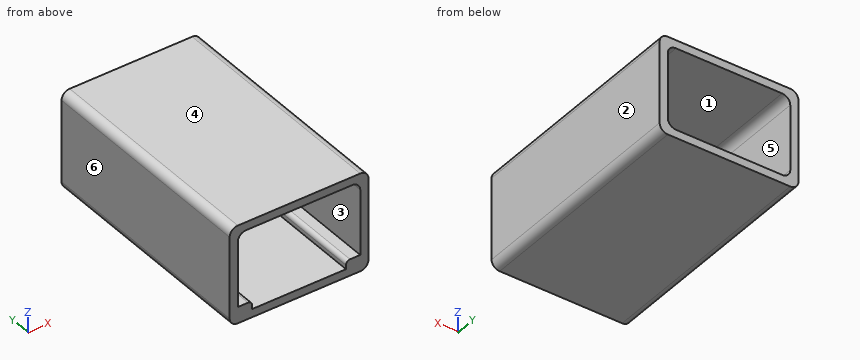
from build123d import *

# Parameters (mm, degrees)
BOSS_EXTRUDE4_DEPTH = 57
BOSS_EXTRUDE5_DEPTH = 51


with BuildPart() as part:
    # Sketch8 → Boss-Extrude4 (new body)
    with BuildSketch(Plane(origin=(0, 58, 0), x_dir=(1, 0, 0), z_dir=(0, 1, 0))):
        with BuildLine():
            Line((-15, -12), (15, -12))
            ThreePointArc((15, -12), (16.414213562, -11.414213562), (17, -10))
            Line((17, -10), (17, 10))
            ThreePointArc((17, 10), (16.414213562, 11.414213562), (15, 12))
            Line((15, 12), (-15, 12))
            ThreePointArc((-15, 12), (-16.414213562, 11.414213562), (-17, 10))
            Line((-17, 10), (-17, -10))
            ThreePointArc((-17, -10), (-16.414213562, -11.414213562), (-15, -12))
        make_face()
        with BuildLine():
            Line((-13, -10), (13, -10))
            ThreePointArc((13, -10), (14.414213562, -9.414213562), (15, -8))
            Line((15, -8), (15, 8))
            ThreePointArc((15, 8), (14.414213562, 9.414213562), (13, 10))
            Line((13, 10), (-13, 10))
            ThreePointArc((-13, 10), (-14.414213562, 9.414213562), (-15, 8))
            Line((-15, 8), (-15, -8))
            ThreePointArc((-15, -8), (-14.414213562, -9.414213562), (-13, -10))
        make_face(mode=Mode.SUBTRACT)
    extrude(amount=BOSS_EXTRUDE4_DEPTH)

    # Sketch11 → Boss-Extrude5 (add)
    with BuildSketch(Plane(origin=(0, 58, 0), x_dir=(1, 0, 0), z_dir=(0, 1, 0))):
        with BuildLine():
            Line((15, 8), (12.5, 8))
            ThreePointArc((12.5, 8), (11.792893219, 8.292893219), (11.5, 9))
            Line((11.5, 9), (11.5, 10))
            Line((11.5, 10), (15, 10))
            Line((15, 10), (15, 8))
        make_face()
        with BuildLine():
            Line((-11.5, 10), (-15, 10))
            Line((-15, 10), (-15, 8))
            Line((-15, 8), (-12.5, 8))
            ThreePointArc((-12.5, 8), (-11.792893219, 8.292893219), (-11.5, 9))
            Line((-11.5, 9), (-11.5, 10))
        make_face()
    extrude(amount=BOSS_EXTRUDE5_DEPTH)


solid = part.part
The model under review builds one solid part; all positions refer to its coordinate system, in mm. Face numbers are marked on the shaded views. A direction names the side the tool comes from. Give positions to 0.01 mm unless a question says otherwise; leave off trailing zeros. Order: outer loops, then holes, each group sorted by start corner. A loop starts at its lowest first (then second) coordinate and runs counter-clockwise, first axis right, second up. Notation, with made-up numbers: M 74,-5 L 112,-5 A23 ccw 112,17 Z; hole C -36,13.5 d5. An arc over 180 degrees is marked long. One line per question, with ' | ' between items. Start each with the question number.
1) Consider section C-C, the plane z = -2.5. Give the boundary of the cut face in (x, y).
2) For the marked faces 5 and 6, list the 3-axis set-ups (+Z, -Z, +X, -X, +Y, -Y) from which the entire face can be reached by the end or side of a thin tool; tool diameter is ignored.
3) Mouldability with a two-part tool opening along X and no side actions: class the marked faces 1, 2, 3 and 4 as pulls with the +X half, pulls with the -X half, needs draft (parallel to the pull), parting line crosses it, or undercut.
4) Clearance check with flat-ended pins moving along their axes: P1, Ø3, axis at x = 10, z = 8, coming from the +Y side; P2, Ø1, axis at x = -13.5, z = -9, coming from the +Y side. State where each tip first meets the part, or that it passes through.
5) Consider section B-B, the plane y = 72.5. Give the boundary of the cut face in (x, z).
6) Consider section A-A, the plane x = -0.5. Give the boundary of the cut face in (y, z).
7) Wall thickness on L1, parallel to X at y = 105.5, z = 3.5; L2, parallel to Z at x = -3, y = 72; L3, parallel to Z at x = 13, y = 83.5: over which ranges is each line inside the solid? List them lowest first. Write a range as from..to.
Found:
1) outline: M -17,58 L -15,58 L -15,115 L -17,115 Z; M 15,58 L 17,58 L 17,115 L 15,115 Z
2) face 5: +Y, -Y | face 6: +Z, -Z, -X, +Y, -Y
3) face 1: undercut | face 2: pulls with the +X half | face 3: undercut | face 4: needs draft
4) P1: passes through | P2: stops at y = 109
5) outline: M -17,-10 A2 ccw -15,-12 L 15,-12 A2 ccw 17,-10 L 17,10 A2 ccw 15,12 L -15,12 A2 ccw -17,10 Z; hole M -15,-8 L -12.5,-8 A1 cw -11.5,-9 L -11.5,-10 L 11.5,-10 L 11.5,-9 A1 cw 12.5,-8 L 15,-8 L 15,8 A2 ccw 13,10 L -13,10 A2 ccw -15,8 Z
6) outline: M 58,-12 L 115,-12 L 115,-10 L 58,-10 Z; M 58,10 L 115,10 L 115,12 L 58,12 Z
7) L1: x = -17..-15, 15..17 | L2: z = -12..-10, 10..12 | L3: z = -12..-8, 10..12
